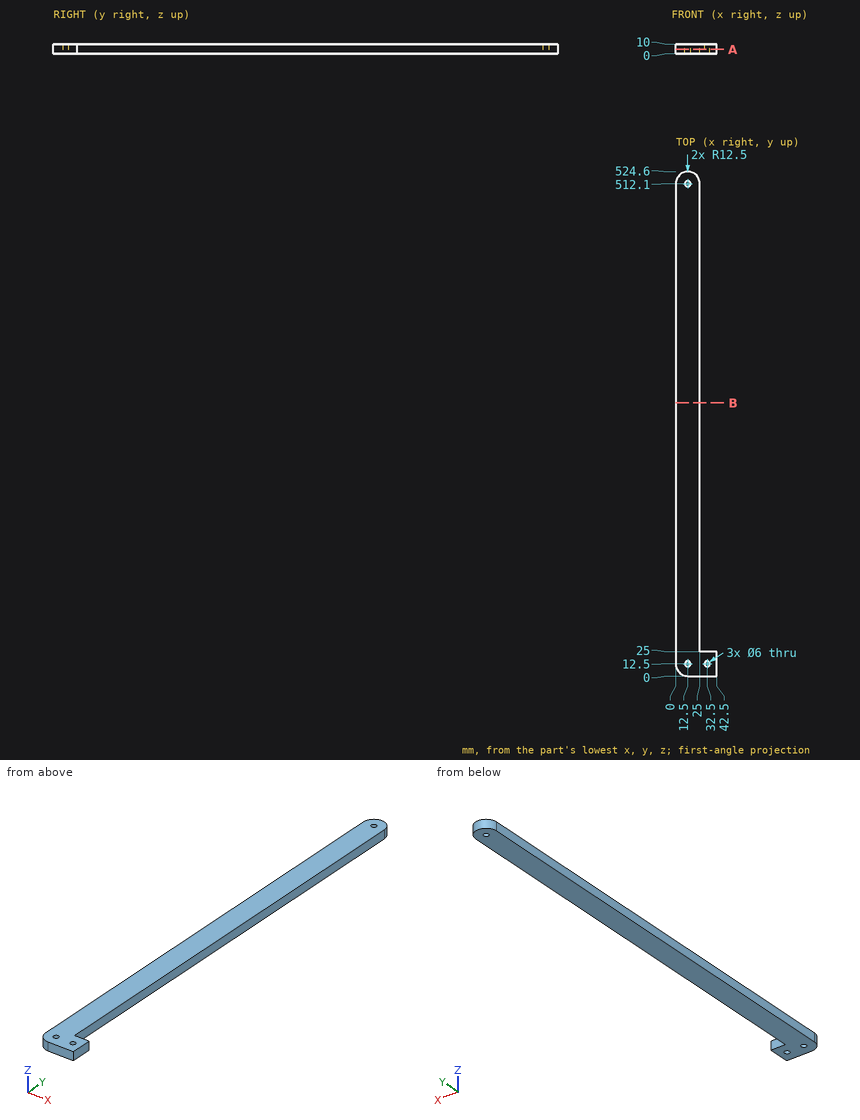
For this review, use the dimensioned drawing (mm, ordinates from the lowest corner) and the shaded views. Give positions to 0.01 mm unless a question says otherwise; leave off trailing zeros. Loops run counter-clockwise (first coordinate to the right, second up) from the corner with the lowest first, then second, coordinate; pieces in that order, holes last.
Item 1: Take a section at B-B, the plane y = 284. State the section outline as (x, z) points, and give its area (3 significant figures).
Item 2: Take a section at A-A, the plane z = 4.5. State the section outline as (x, y) points, and give its area (3 significant figures).
Item 3: Insertion check: pin 1 (3.5 mm diameter, centred on x = 12.5, y = 12.5, fed in from -Z); pin 2 (1.5 mm diameter, centred on y = 281, z = 4, fed in from +X); pin 3 (5 mm diameter, centred on x = 5.5, z = 7, fed in from +Y). Each pin has a flat end and moves straight along its axis. Give the tip position at first contact, or say it passes through.
Item 4: For line 1 along X through (y, z) = (12.5, 4); line 2 along Y through (x, z) = (32.5, 6); line 3 along Y through (x, z) = (13.5, 3), list the stretches that pass through material, from the lowest coordinate up.
Calculated:
1. outline: (0, 0) - (25, 0) - (25, 10) - (0, 10) - close
1. area: 250 mm2
2. outline: (0, 12.5) arc R12.5 ccw to (12.5, 0) - (42.5, 0) - (42.5, 25) - (25, 25) - (25, 512.1) arc R12.5 ccw to (0, 512.1) - close; hole circle Ø6 at (12.5, 12.5); hole circle Ø6 at (12.5, 512.1); hole circle Ø6 at (32.5, 12.5)
2. area: 13,400 mm2
3. pin 1: passes through
3. pin 2: stops at x = 25
3. pin 3: stops at y = 523.76
4. line 1: x = 0 to 9.5, 15.5 to 29.5, 35.5 to 42.5
4. line 2: y = 0 to 9.5, 15.5 to 25
4. line 3: y = 0 to 9.67, 15.33 to 509.27, 514.93 to 524.56
